Source: CAD feature listing. Evaluate the final solid. Frame: model axes, mm. Face numbers are marked on the shaded views. A direction names the side the tool comes from. Coordinates: 2 decimals unless noted, no trailing zeros. Write each loop counter-clockwise with the first axis right and the second up, starting at its lowest first coordinate (ties: lowest second). Pieces come first, ordered by that corner, then holes. Notation, with made-up numbers: (69.25, 53.5) -> (124.25, 53.5) arc R16 ccw to (124.25, 69.5) -> close; hole circle Ø2 at (-5, -29.5). An arc over 180 degrees is marked (long way). Write item = value, one per line.
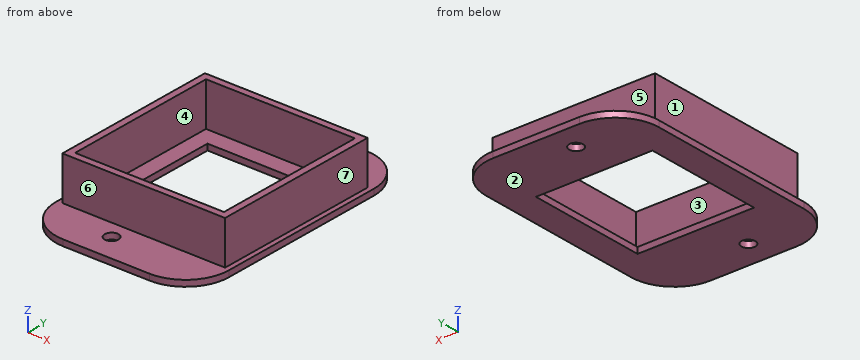
from build123d import *

# Parameters (mm, degrees)
F0_W     = 40
F0_H     = 60
F1_DEPTH = 1.4
F2_W     = 37.7
F2_H     = 39.3
F2_W_2   = 34.5
F2_H_2   = 36.1
F3_DEPTH = 10
F4_R     = 1.6
F4_W     = 27
F4_H     = 28
F5_DEPTH = 1.401
F6_R     = 10


with BuildPart() as f1:
    # F0 (on Top) → F1 (new body)
    with BuildSketch(Plane.XY):
        Rectangle(F0_W, F0_H)
    extrude(amount=F1_DEPTH)

    # F2 (on face) → F3 (join)
    with BuildSketch(Plane.XY.offset(1.4)):
        Rectangle(F2_W, F2_H)
        Rectangle(F2_W_2, F2_H_2, mode=Mode.SUBTRACT)
    extrude(amount=F3_DEPTH)

    # F4 (on face) → F5 (cut, through all)
    with BuildSketch(Plane.XY.offset(1.4)):
        with Locations((-4, 23.75)):
            Circle(F4_R)
        with Locations((-4, -23.75)):
            Circle(F4_R)
        Rectangle(F4_W, F4_H)
    extrude(amount=-F5_DEPTH, mode=Mode.SUBTRACT)

    # F6
    f6_edges = [f1.edges().sort_by_distance(p)[0] for p in [
        (-20, -30, 0.7),
        (20, -30, 0.7),
        (20, 30, 0.7),
        (-20, 30, 0.7),
    ]]
    fillet(f6_edges, radius=F6_R)


solid = f1.part
1) Cut plane D-D, the plane y = 23.75. Output: boundary loops of the cut face in (x, z), and give its area (3 significant figures).
Answer block:
outline = (-19.27, 0) -> (-5.6, 0) -> (-5.6, 1.4) -> (-19.27, 1.4) -> close; (-2.4, 0) -> (19.27, 0) -> (19.27, 1.4) -> (-2.4, 1.4) -> close
area = 49.5 mm2
2) Cut plane C-C, the plane x = -8. Output: boundary loops of the cut face in (y, z), and give its area (3 significant figures).
Answer block:
outline = (-30, 0) -> (-14, 0) -> (-14, 1.4) -> (-18.05, 1.4) -> (-18.05, 11.4) -> (-19.65, 11.4) -> (-19.65, 1.4) -> (-30, 1.4) -> close; (14, 0) -> (30, 0) -> (30, 1.4) -> (19.65, 1.4) -> (19.65, 11.4) -> (18.05, 11.4) -> (18.05, 1.4) -> (14, 1.4) -> close
area = 76.8 mm2
3) First-contact query: pin 1 Ø4 at (x, y) = (-4, -23.75) entering from +Z; pin 2 Ø1 at (y, z) = (-14.5, 8) entering from +X; pin 3 Ø8 at (x, y) = (7.5, 0) entering from -Z; pin 4 Ø5 at (x, z) = (1, 7.5) entering from -Y. Flat tips, straight axial feed; report the tip coordinate or a pass-through.
Answer block:
pin_1 = 1.4
pin_2 = 18.85
pin_3 = through
pin_4 = -19.65
4) Pull-direction query (X, two-part tool) for the marked faces 1, 2 and 3; classes: +X half, -X half, draft (parallel to the pull), parting line (faces both ways), or undercut.
Answer block:
face_1 = -X half
face_2 = draft
face_3 = undercut
5) Reachability of the marked faces 4, 5, 6 and 7 from +Z, -Z, +X, -X, +Y, -Y: full face, straight path, thin tool, end or side. Return the list, or none.
Answer block:
face_4 = +Z
face_5 = +Z, +X, -X, +Y
face_6 = +Z, +X, -X, -Y
face_7 = +Z, +X, +Y, -Y
6) Cut plane B-B, the plane x = -4. Output: boundary loops of the cut face in (y, z).
Answer block:
outline = (-30, 0) -> (-25.35, 0) -> (-25.35, 1.4) -> (-30, 1.4) -> close; (-22.15, 0) -> (-14, 0) -> (-14, 1.4) -> (-18.05, 1.4) -> (-18.05, 11.4) -> (-19.65, 11.4) -> (-19.65, 1.4) -> (-22.15, 1.4) -> close; (14, 0) -> (22.15, 0) -> (22.15, 1.4) -> (19.65, 1.4) -> (19.65, 11.4) -> (18.05, 11.4) -> (18.05, 1.4) -> (14, 1.4) -> close; (25.35, 0) -> (30, 0) -> (30, 1.4) -> (25.35, 1.4) -> close
7) Material intervals for probe 1 along Y at (x, z) = (-4, 0.7); probe 2 along Y at (x, z) = (-8, 7.5); probe 3 along X at (y, z) = (-2, 5.25), sorted ascending. Write a range as [from, to].
Answer block:
probe_1 = [-30, -25.35], [-22.15, -14], [14, 22.15], [25.35, 30]
probe_2 = [-19.65, -18.05], [18.05, 19.65]
probe_3 = [-18.85, -17.25], [17.25, 18.85]
8) Cut plane A-A, the plane y = -3.5. Output: boundary loops of the cut face in (x, z), and give its area (3 significant figures).
Answer block:
outline = (-20, 0) -> (-13.5, 0) -> (-13.5, 1.4) -> (-17.25, 1.4) -> (-17.25, 11.4) -> (-18.85, 11.4) -> (-18.85, 1.4) -> (-20, 1.4) -> close; (13.5, 0) -> (20, 0) -> (20, 1.4) -> (18.85, 1.4) -> (18.85, 11.4) -> (17.25, 11.4) -> (17.25, 1.4) -> (13.5, 1.4) -> close
area = 50.2 mm2
